The listing builds one solid part. Answer for the finished solid, in the listing's coordinates (mm). Face numbers are marked on the shaded views. A direction names the side the tool comes from. Round coordinates to 2 decimals unless told otherwise and drop trailing zeros. Write each loop counter-clockwise with the first axis right and the second up, starting at its lowest first coordinate (ties: lowest second). Pieces come first, ordered by that corner, then holes.
(1) Find the intervals of material crossed by probe 1 along Z at (x, y) = (-12.5, 0); probe 2 along X at (y, z) = (-2.75, 1); probe 3 along Z at (x, y) = (4, -0.5), in increasing order.
(2) For the marked faces 1, 2 and 3, determine the directions among +Z, -Z, +X, -X, +Y, -Y from which every point of the face is accessible in a straight line to the end or side of a thin tool.
(3) Each of these flat-tipped pins is pushed along its axis until it touches: pin 1 Ø1 at (x, y) = (-7.5, 1) entering from +Z; pin 2 Ø3 at (x, z) = (-12, -1) entering from +Y. Where does it stop, or does it pass through?
(4) A cutting plane is placed at D-D, the plane x = -1.5. Give the vertices of the cut face in (y, z).
(5) A cutting plane is placed at C-C, the plane x = -12.5. Give the vertices of the cut face in (y, z), and give its area (3 significant figures).
(6) A cutting plane is placed at A-A, the plane y = 0. Give the vertices of the cut face in (x, z).
from build123d import *

# Parameters (mm, degrees)
SKETCH1_W = 5.5
SKETCH1_H = 1.5


with BuildPart() as part:
    # Sketch1 → Revolve1 (revolve)
    with BuildSketch(Plane.XY):
        Polygon((-10, 0), (10, 0), (10, 1.5), (10, 3.33), (-10, 3.33), (-10, 1.5), align=None)
        with Locations((-12.75, 0.75)):
            Rectangle(SKETCH1_W, SKETCH1_H)
        with Locations((12.75, 0.75)):
            Rectangle(SKETCH1_W, SKETCH1_H)
    revolve(axis=Axis((-15.5, 0, 0), (1, 0, 0)))


solid = part.part
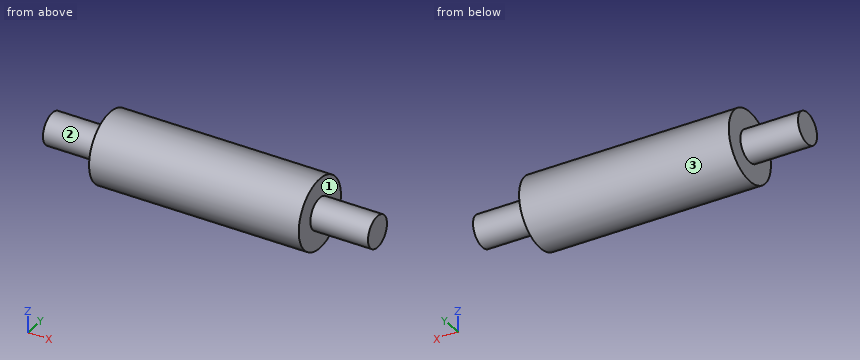
Solutions:
1. probe 1: z = -1.5 to 1.5
1. probe 2: x = -10 to 10
1. probe 3: z = -3.29 to 3.29
2. face 1: +X
2. face 2: -X
2. face 3: +X, -X
3. pin 1: stops at z = 3.29
3. pin 2: stops at y = 1.5
4. outline: circle Ø6.66 at (0, 0)
5. outline: circle Ø3 at (0, 0)
5. area: 7.07 mm2
6. outline: (-15.5, -1.5) - (-10, -1.5) - (-10, -3.33) - (10, -3.33) - (10, -1.5) - (15.5, -1.5) - (15.5, 1.5) - (10, 1.5) - (10, 3.33) - (-10, 3.33) - (-10, 1.5) - (-15.5, 1.5) - close
